```python
from build123d import *

# Parameters (mm, degrees)
F1_DEPTH = 6.35
F2_R     = 12.7
F3_DEPTH = 12.7
F4_R     = 6.35
F5_DEPTH = 19.05


with BuildPart() as f1:
    # F0 (on Top) → F1 (new body)
    with BuildSketch(Plane.XY):
        with BuildLine():
            ThreePointArc((0, 25.4), (-12.7, 12.7), (0, 0))
            Line((0, 0), (19.05, 0))
            Line((19.05, 0), (25.4, 12.7))
            Line((25.4, 12.7), (25.4, 25.4))
            Line((25.4, 25.4), (0, 25.4))
        make_face()
    extrude(amount=F1_DEPTH)

    # F2 (on face) → F3 (join)
    with BuildSketch(Plane.XY.offset(6.35)):
        with Locations((0, 12.7)):
            Circle(F2_R)
    extrude(amount=F3_DEPTH)

    # F4 (on face) → F5 (cut)
    with BuildSketch(Plane.XY.offset(19.05)):
        with Locations((0, 12.7)):
            Circle(F4_R)
    extrude(amount=-F5_DEPTH, mode=Mode.SUBTRACT)


solid = f1.part
```
Input: part model. Units: mm. Frame: model coordinates. A direction names the side the tool comes from. Give positions to 0.01 mm unless a question says otherwise; leave off trailing zeros. Order: outer loops, then holes, each group sorted by start corner. A loop starts at its lowest first (then second) coordinate and runs counter-clockwise, first axis right, second up.
1. Cut plane D-D (x = 2). Return loops of the section in (y, z).
Computed:
outline: (0, 0) - (6.67, 0) - (6.67, 19.05) - (0.16, 19.05) - (0.16, 6.35) - (0, 6.35) - close; (18.73, 0) - (25.4, 0) - (25.4, 6.35) - (25.24, 6.35) - (25.24, 19.05) - (18.73, 19.05) - close
2. Cut plane C-C (z = 11.25). Return loops of the section in (x, y), and give its area (3 significant figures).
Computed:
outline: circle Ø25.4 at (0, 12.7); hole circle Ø12.7 at (0, 12.7)
area: 380 mm2
3. Line query: probe 1 along Y at (x, z) = (0, 15); probe 2 along Z at (x, y) = (19, 13.25); probe 3 along X at (y, z) = (15, 2.5). Output: solid intervals per line, ascending.
Computed:
probe 1: y = 0 to 6.35, 19.05 to 25.4
probe 2: z = 0 to 6.35
probe 3: x = -12.49 to -5.92, 5.92 to 25.4
4. Draft query along X for faces 3 (the face through (10, 13, 0)), 4 (the face through (3.414, 18.054, 9.658)), 5 (the face through (-12.688, 13.258, 11.508)). Return one class per face: released by +X, released by -X, zero draft, split by the parting line, or undercut.
Computed:
face 3: zero draft
face 4: undercut
face 5: split by the parting line
5. Cut plane B-B (x = 9). Return loops of the section in (y, z), and give its area (3 significant figures).
Computed:
outline: (0, 0) - (25.4, 0) - (25.4, 6.35) - (21.66, 6.35) - (21.66, 19.05) - (3.74, 19.05) - (3.74, 6.35) - (0, 6.35) - close
area: 389 mm2
6. Pin query (flat end, axial travel): pin 1 Ø1 at (y, z) = (16.5, 11.5) entering from -X; pin 2 Ø1 at (y, z) = (8.5, 13) entering from +X; pin 3 Ø3 at (y, z) = (22, 9.5) entering from -X. Return the tip coordinate at first contact, or that it passes through.
Computed:
pin 1: stops at x = -12.26
pin 2: stops at x = 12.15
pin 3: stops at x = -10.02
7. Set-up query: faces 1 (the face through (3, 19, 19.05)), 2 (the face through (15, 13, 6.35)). Return all of +Z, -Z, +X, -X, +Y, -Y with unobstructed straight access to the full face (end or side cutting, diameter ignored); none if empty.
Computed:
face 1: +Z, +X, -X, +Y, -Y
face 2: +Z, +X
8. Cut plane A-A (y = 15.5). Return loops of the section in (x, z).
Computed:
outline: (-12.39, 0) - (-5.7, 0) - (-5.7, 19.05) - (-12.39, 19.05) - close; (5.7, 0) - (25.4, 0) - (25.4, 6.35) - (12.39, 6.35) - (12.39, 19.05) - (5.7, 19.05) - close
